Design review of the part built by this model. Coordinates are the model's own, in mm. A direction names the side the tool comes from. Coordinates: 2 decimals unless noted, no trailing zeros. Loops run counter-clockwise (first coordinate to the right, second up) from the corner with the lowest first, then second, coordinate; pieces in that order, holes last. Notation, with made-up numbers: (27.5, 64) - (69.5, 64) arc R18 cw to (69.5, 98) - close; hole circle Ø5 at (61, -7). An arc over 180 degrees is marked (long way). Answer in a Markdown table with one row per item. Add a question column.
(1) We need section A-A, the plane y = -24. Write out the cut boundary in (x, z).
(2) For faces 1 (the face through (-35, -8, 8)), 2 (the face through (-14, -39, 48.148)), list the 3-axis set-ups (+Z, -Z, +X, -X, +Y, -Y) from which the entire face can be reached by the end or side of a thin tool; tool diameter is ignored.
(3) To check wall thickness, follow L1, parallel to Z at x = 560, y = -56.5; L2, parallel to Y at x = -574.5, z = 29; L3, parallel to X at y = -7, z = -16.5. State the ranges of each line that lie inside material, in increasing order. Write a range as [from, to].
(4) We need section B-B, the plane x = -550. Write out the cut boundary in (y, z).
(5) The part is to be moulded in two halves that separate along Z. For faces 3 (the face through (-35, -72, 8)), 4 (the face through (-687.835, -75, 9)), 5 (the face through (615.825, -74.996, 7.588)), say which applies: released by +Z, released by -Z, zero draft, split by the parting line, or undercut.
(6) Clearance check with flat-ended pins moving along their axes: pin 1 (8 mm diameter, centred on y = -47, z = -23.5, fed in from +X); pin 2 (19 mm diameter, centred on x = -261.5, z = -2, fed in from +Y). State where each tip first meets the part, or that it passes through.
from build123d import *

# Parameters (mm, degrees)
F1_DEPTH = 80
F2_W     = 64
F2_H     = 64
F3_DEPTH = 1330
F4_D     = 26


with BuildPart() as f1:
    # F0 (on Front) → F1 (new body)
    with BuildSketch(Plane.XZ):
        Polygon((642.1647218585, 48.1479109465), (-687.8352781415, 48.1479109465), (-687.8352781415, -31.8520890535), (590.2121144027, -31.8520890535), align=None)
    extrude(amount=F1_DEPTH)

    # F2 (on face) → F3 (cut)
    with BuildSketch(Plane(origin=(-687.8352781415, 0, 0), x_dir=(0, -1, 0), z_dir=(-1, 0, 0))):
        with Locations((40, 8.1479109465)):
            Rectangle(F2_W, F2_H)
    extrude(amount=-F3_DEPTH, mode=Mode.SUBTRACT)

    # F4 (through all)
    with Locations(Plane(origin=(0, 0, 0), x_dir=(1, 0, 0), z_dir=(0, 1, 0))):
        with Locations((-652.8352781415, -8.1479109465)):
            Hole(F4_D / 2)


solid = f1.part
Responses:
| question | item | result |
|---|---|---|
| 1 | outline | (-687.84, -31.85) - (590.21, -31.85) - (595.41, -23.85) - (-687.84, -23.85) - close; (-687.84, 40.15) - (636.97, 40.15) - (642.16, 48.15) - (-687.84, 48.15) - close |
| 2 | face 1 | +X, -X |
| 2 | face 2 | +Z, +X, -X, +Y, -Y |
| 3 | L1 | z = [-31.85, -23.85], [40.15, 48.15] |
| 3 | L2 | y = [-80, -72], [-8, 0] |
| 3 | L3 | x = [-687.84, 600.18] |
| 4 | outline | (-80, -31.85) - (0, -31.85) - (0, 48.15) - (-80, 48.15) - close; hole (-72, -23.85) - (-8, -23.85) - (-8, 40.15) - (-72, 40.15) - close |
| 5 | face 3 | undercut |
| 5 | face 4 | zero draft |
| 5 | face 5 | released by -Z |
| 6 | pin 1 | stops at x = 595.41 |
| 6 | pin 2 | stops at y = 0 |
